Geometry: final body of the model. Coordinates: model frame, mm. A direction names the side the tool comes from. Coordinates: 2 decimals unless noted, no trailing zeros. Order: outer loops, then holes, each group sorted by start corner. A loop starts at its lowest first (then second) coordinate and runs counter-clockwise, first axis right, second up. Notation, with made-up numbers: (38.25, -36.75) -> (95.25, -36.75) arc R21 cw to (95.25, -3.75) -> close; hole circle Ø3 at (64, -37). An arc over 180 degrees is marked (long way). Answer in a Markdown table with one row per item. Add a question column.
1) Section query B-B on x = 4. Return the cut outline in (y, z).
2) Section query A-A on z = 13.75. Count the separate pieces of the cut face and the enclosed holes in it, then the cut area to 3 significant figures.
3) Section query D-D on y = -25.5. Return the cut outline in (x, z), then the cut area to 3 significant figures.
4) Contact query for flat-ended pins moving along their axis: P1, Ø6.5, axis at x = 35, y = 0, coming from the +Z side; P2, Ø3, axis at y = -48.5, z = 8, coming from the +X side; P3, Ø11.5, axis at x = -31.5, y = -20.5, coming from the +Z side; P4, Ø5.5, axis at y = -67.5, z = 7.5, coming from the -X side. Output: stop coordinate, or through.
5) Pull-direction query (X, two-part tool) for faces 1 (the face through (-27, 19.604, 2)), 2 (the face through (32.214, -68, 12)), 3 (the face through (-38.938, -46, 14)); classes: +X half, -X half, draft (parallel to the pull), parting line (faces both ways), or undercut.
6) Set-up query: faces 4 (the face through (28, 9.425, 2)), 5 (the face through (0, -84.428, 3)), 6 (the face through (33, -28.478, 11)), 7 (the face through (-32, -29.682, 12)), 8 (the face through (0, -42, 0)). Return all of +Z, -Z, +X, -X, +Y, -Y with unobstructed straight access to the full face (end or side cutting, diameter ignored); none if empty.
7) Ray query, line 1 (Y direction, x = -37, z = 6.5); line 2 (Y direction, x = -30, z = 8.5); line 3 (Y direction, x = -22.5, z = 3.75). Return the intervals inside material, ascending. Write a range as from..to.
8) Section query C-C on y = -77. Return the cut outline in (x, z), then the cut area to 3 significant figures.
```python
from build123d import *

# Parameters (mm, degrees)
BASE_SEGUIDOR_DEPTH        = 5
RESIZE_BASE_BY             = 10.718934909
RESIZE_BASE_2_BY           = 6.304160727
MOVER_START                = -87.004758572
MOVER_FACE10_OUTLINE_W     = 90.28944226
MOVER_FACE10_OUTLINE_H     = 5
MOVER_FACE10_DEPTH         = 4.845951812
ESBO_O27_W                 = 5.735972996
ESBO_O27_H                 = 5.741390801
ESBO_O27_W_2               = 5.190846063
BASE_ENGERENAGEM_DEPTH     = 18
ESBO_O18_R                 = 24.046540625
ESBO_O18_R_2               = 21.423073694
RESSALTO_EXTRUS_O11_DEPTH  = 5
ESBO_O22_W                 = 57.28918899
ESBO_O22_H                 = 33.028358432
CORTE_EXTRUS_O2_DEPTH      = 4
RESSALTO_EXTRUS_O12_DEPTH  = 15
ESBO_O26_W                 = 5.982118077
ESBO_O26_H                 = 10.002665269
CORTE_EXTRUS_O3_DEPTH      = 64
ESBO_O6_W                  = 25.148684125
ESBO_O6_H                  = 14.153877123
ESBO_O6_W_2                = 25.424126456
RESSALTO_EXTRUS_O10_DEPTH  = 14
ESBO_O19_W                 = 12.585961191
ESBO_O19_H                 = 12.087029767
CORTE_EXTRUS_O1_DEPTH      = 92
ESBO_O4_W                  = 21.689466083
ESBO_O4_H                  = 21.567386105
PCB_BURACOS_DEPTH          = 4
ESBO_O2_W                  = 71.017341725
ESBO_O2_H                  = 21.492860186
SENSOR_INFRA_ENCAIXE_DEPTH = 3
ESBO_O9_W                  = 67.154361664
ESBO_O9_H                  = 7.082446002
FURO_SENSOR_DEPTH          = 10


# Read off the part's stored shape, not the designer's step: Mover face10
with BuildPart() as part:
    # Esboço1 → base_seguidor (new body)
    with BuildSketch(Plane.XY):
        Polygon((-44.67348187, 40.715072084), (-44.67348187, 19.603553226), (-9.047793796, 19.603553226), (-9.047793796, 9.424785205), (-44.67348187, 9.424785205), (-44.67348187, -71.439871851), (45.61596039, -71.439871851), (45.61596039, 9.424785205), (10.178768021, 9.424785205), (10.178768021, 19.603553226), (45.61596039, 19.603553226), (45.61596039, 40.715072084), align=None)
    extrude(amount=BASE_SEGUIDOR_DEPTH)

    # resize_base: a face moved outward by 10.718935
    extrude(part.faces().sort_by_distance((0.47123926, -71.439871851, 2.5))[0], amount=RESIZE_BASE_BY, dir=(0, -1, 0))

    # resize_base_2: a face moved outward by 6.304161
    extrude(part.faces().sort_by_distance((0.47123926, 40.715072084, 2.5))[0], amount=RESIZE_BASE_2_BY, dir=(0, 1, 0))

    # Mover face10 outline → Mover face10 (add)
    with BuildSketch(Plane(origin=(0, 0, 0), x_dir=(1, 0, 0), z_dir=(0, 1, 0)).offset(MOVER_START)):
        with Locations((0.47123926, -2.5)):
            Rectangle(MOVER_FACE10_OUTLINE_W, MOVER_FACE10_OUTLINE_H)
    extrude(amount=MOVER_FACE10_DEPTH)

    # Esboço27 → base_engerenagem (add)
    with BuildSketch(Plane.XY.offset(5)):
        with Locations((-41.805495372, -46.264886582)):
            Rectangle(ESBO_O27_W, ESBO_O27_H)
        with Locations((43.020537359, -46.264886582)):
            Rectangle(ESBO_O27_W_2, ESBO_O27_H)
    extrude(amount=BASE_ENGERENAGEM_DEPTH)

    # Esboço18 → Ressalto-extrusão11 (add)
    with BuildSketch(Plane.XY.offset(5)):
        with Locations((-0.274583628, -109.638466508)):
            Circle(ESBO_O18_R)
        with Locations((-0.274583628, -109.638466508)):
            Circle(ESBO_O18_R_2, mode=Mode.SUBTRACT)
    extrude(amount=-RESSALTO_EXTRUS_O11_DEPTH)

    # Esboço22 → Corte-extrusão2 (cut)
    with BuildSketch(Plane.XY.offset(5)):
        with Locations((0.373700248, -67.914265776)):
            Rectangle(ESBO_O22_W, ESBO_O22_H)
    extrude(amount=-CORTE_EXTRUS_O2_DEPTH, mode=Mode.SUBTRACT)

    # Esboço24 → Ressalto-extrusão12 (add)
    with BuildSketch(Plane.XY.offset(5)):
        Polygon((-28.270894247, -51.40008656), (-30.823687143, -48.847293665), (-30.823687143, -87.004758572), (-28.270894247, -84.428444992), align=None)
        Polygon((29.018294743, -51.40008656), (32.214208361, -49.269582228), (32.214208361, -87.004758572), (29.018294743, -84.428444992), align=None)
    extrude(amount=RESSALTO_EXTRUS_O12_DEPTH)

    # Esboço26 → Corte-extrusão3 (cut)
    with BuildSketch(Plane(origin=(32.214208361, 0, 0), x_dir=(0, 0, -1), z_dir=(1, 0, 0))):
        with Locations((-7.991059039, -68.064198105)):
            Rectangle(ESBO_O26_W, ESBO_O26_H)
    extrude(amount=-CORTE_EXTRUS_O3_DEPTH, mode=Mode.SUBTRACT)

    # Esboço6 → Ressalto-extrusão10 (add)
    with BuildSketch(Plane.XY.offset(5)):
        with Locations((33.131077051, -22.60517657)):
            Rectangle(ESBO_O6_W, ESBO_O6_H)
        with Locations((-31.871959919, -22.60517657)):
            Rectangle(ESBO_O6_W_2, ESBO_O6_H)
    extrude(amount=RESSALTO_EXTRUS_O10_DEPTH)

    # Esboço19 → Corte-extrusão1 (cut)
    with BuildSketch(Plane.ZY.offset(44.67348187)):
        with Locations((11.292980596, -22.434877547)):
            Rectangle(ESBO_O19_W, ESBO_O19_H)
    extrude(amount=-CORTE_EXTRUS_O1_DEPTH, mode=Mode.SUBTRACT)

    # Esboço4 → pcb_buracos (cut)
    with BuildSketch(Plane.XY.offset(5)):
        Polygon((-15.516819289, 7.573140349), (16.485994782, 7.741548684), (16.485994782, -47.664793519), (-14.412520449, -47.664793519), align=None)
        with Locations((33.019910346, -2.978526461)):
            Rectangle(ESBO_O4_W, ESBO_O4_H)
    extrude(amount=-PCB_BURACOS_DEPTH, mode=Mode.SUBTRACT)

    # Esboço2 → sensor_infra_encaixe (cut)
    with BuildSketch(Plane.XY.offset(5)):
        with Locations((0.47123926, 36.272802718)):
            Rectangle(ESBO_O2_W, ESBO_O2_H)
    extrude(amount=-SENSOR_INFRA_ENCAIXE_DEPTH, mode=Mode.SUBTRACT)

    # Esboço9 → furo_sensor (cut)
    with BuildSketch(Plane.XY.offset(2)):
        with Locations((0.411915335, 38.971892304)):
            Rectangle(ESBO_O9_W, ESBO_O9_H)
    extrude(amount=-FURO_SENSOR_DEPTH, mode=Mode.SUBTRACT)


solid = part.part
```
Result:
| question | item | result |
|---|---|---|
| 1 | outline | (-133.3, 0) -> (-130.63, 0) -> (-130.63, 5) -> (-133.3, 5) -> close; (-88.65, 0) -> (35.43, 0) -> (35.43, 2) -> (25.53, 2) -> (25.53, 5) -> (7.68, 5) -> (7.68, 1) -> (-47.66, 1) -> (-47.66, 5) -> (-51.4, 5) -> (-51.4, 1) -> (-84.43, 1) -> (-84.43, 5) -> (-88.65, 5) -> close; (42.51, 0) -> (47.02, 0) -> (47.02, 2) -> (42.51, 2) -> close |
| 2 | separate pieces | 8 |
| 2 | enclosed holes | 0 |
| 2 | area | 371 mm2 |
| 3 | outline | (-44.67, 0) -> (45.62, 0) -> (45.62, 5) -> (16.49, 5) -> (16.49, 1) -> (-14.86, 1) -> (-14.86, 5) -> (-44.67, 5) -> close; (-44.58, 17.59) -> (-19.16, 17.59) -> (-19.16, 19) -> (-44.58, 19) -> close; (20.56, 17.59) -> (45.71, 17.59) -> (45.71, 19) -> (20.56, 19) -> close |
| 3 | area | 398 mm2 |
| 4 | P1 | z = 1 |
| 4 | P2 | x = 45.62 |
| 4 | P3 | z = 19 |
| 4 | P4 | x = -44.67 |
| 5 | face 1 | draft |
| 5 | face 2 | +X half |
| 5 | face 3 | undercut |
| 6 | face 4 | +Z, -Z, +X |
| 6 | face 5 | +Z |
| 6 | face 6 | +X, -X |
| 6 | face 7 | +Z, +X, -X |
| 6 | face 8 | -Z, +X, -X, +Y, -Y |
| 7 | line 1 | -29.68..-28.48, -16.39..-15.53 |
| 7 | line 2 | -86.17..-73.07, -63.06..-49.67, -29.68..-28.48, -16.39..-15.53 |
| 7 | line 3 | -118.82..-100.46, -87..-84.43, -51.4..9.42, 19.6..25.53 |
| 8 | outline | (-44.67, 0) -> (45.62, 0) -> (45.62, 5) -> (32.21, 5) -> (32.21, 20) -> (29.02, 20) -> (29.02, 1) -> (-28.27, 1) -> (-28.27, 20) -> (-30.82, 20) -> (-30.82, 5) -> (-44.67, 5) -> close |
| 8 | area | 309 mm2 |
